Design review of the part shown in the three views and the two pictorial views. Dimensions are in mm from the part's minimum x, y and z. A direction names the side the tool comes from. Round coordinates to 2 decimals unless told otherwise and drop trailing zeros. Write each loop counter-clockwise with the first axis right and the second up, starting at its lowest first coordinate (ties: lowest second). Pieces come first, ordered by that corner, then holes. Notation, with made-up numbers: (3.5, 40.5) -> (28.5, 40.5) arc R30 cw to (28.5, 72.5) -> close; hole circle Ø2 at (22.25, 20.25). An arc over 180 degrees is marked (long way). Answer as a JSON object with one key per item and string values. Group by question number.
1) Machinability: for the marked faces 4 and 5, which of the approach directions +Z, -Z, +X, -X, +Y, -Y give a long, thin tool a straight path to every point of the face, cutting with its end or side? Answer none if there is none.
2) To check wall thickness, follow probe 1 along Y at (x, z) = (4.5, 1.5); probe 2 along X at (y, z) = (11.5, 4.4). State the ranges of each line that lie inside material, in increasing order. Write a range as [from, to].
3) Mouldability with a two-part tool opening along Y and no side actions: class the marked faces 1, 2 and 3 as pulls with the +Y half, pulls with the -Y half, needs draft (parallel to the pull), parting line crosses it, or undercut.
4) We need section D-D, the plane z = 4.35. Write out the cut boundary in (x, y).
5) We need section B-B, the plane y = 25.25. Write out the cut boundary in (x, z), then the cut area to 3 significant figures.
6) We need section A-A, the plane z = 2.05. Write out the cut boundary in (x, y).
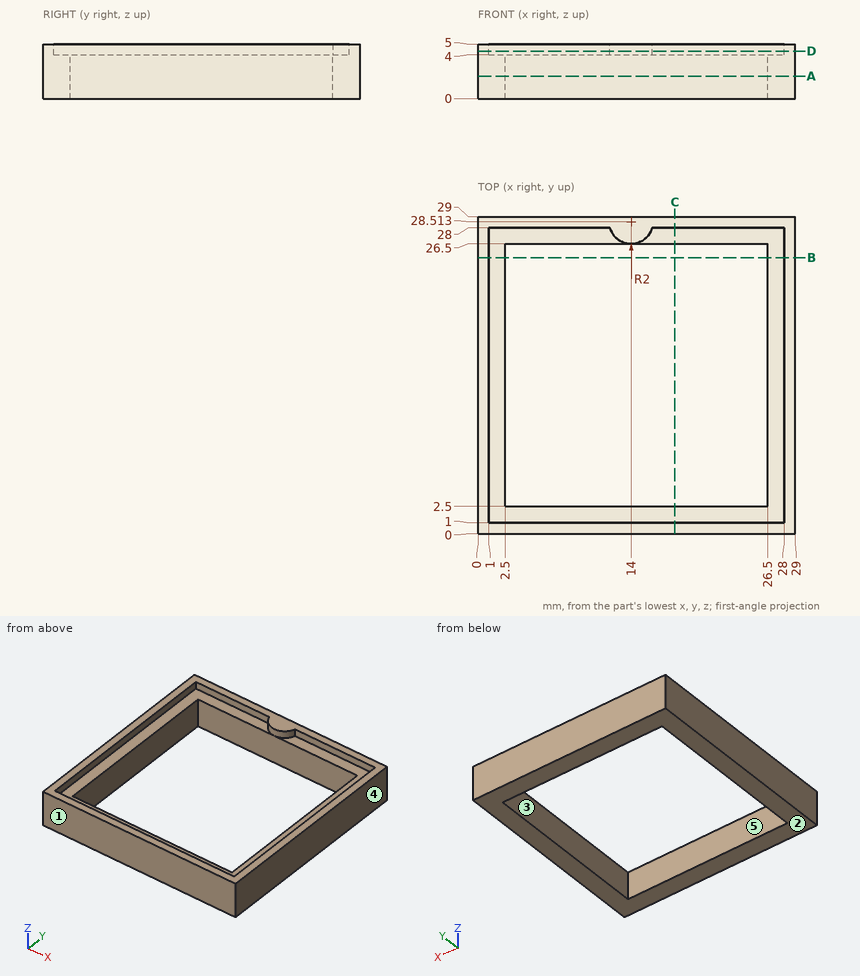
Here are the results:
{
 "1": {"face 4": "+Z, -Z, +X, +Y, -Y", "face 5": "+Z, -Z"},
 "2": {"probe 1": "y = [0, 2.5], [26.5, 29]", "probe 2": "x = [0, 1], [28, 29]"},
 "3": {"face 1": "pulls with the -Y half", "face 2": "needs draft", "face 3": "undercut"},
 "4": {"outline": "(0, 0) -> (29, 0) -> (29, 29) -> (0, 29) -> close; hole (1, 1) -> (28, 1) -> (28, 28) -> (15.93, 28) arc R2 cw to (12.07, 28) -> (1, 28) -> close"},
 "5": {"outline": "(0, 0) -> (2.5, 0) -> (2.5, 4) -> (1, 4) -> (1, 5) -> (0, 5) -> close; (26.5, 0) -> (29, 0) -> (29, 5) -> (28, 5) -> (28, 4) -> (26.5, 4) -> close", "area": "22.0 mm^2"},
 "6": {"outline": "(0, 0) -> (29, 0) -> (29, 29) -> (0, 29) -> close; hole (2.5, 2.5) -> (26.5, 2.5) -> (26.5, 26.5) -> (2.5, 26.5) -> close"}
}
